CAD build for the part. Positions are in the model's coordinates, mm. Give positions to 0.01 mm unless a question says otherwise; leave off trailing zeros. Answer as a JSON object with one key per item and string values.
Autodesk Inventor part; units mm, degrees
ref_plane "C1_XY" through (0, 0, 0) normal (0, 0, 1) x (1, 0, 0)
ref_plane "C1_YZ" through (0, 0, 0) normal (1, 0, 0) x (0, 1, 0)
ref_plane "C1_ZX" through (0, 0, 0) normal (0, 1, 0) x (0, 0, 1)
sketch "Sketch_1" plane through (0, 0, 0) normal (0, 0, 1) x (1, 0, 0)
  line L0 (-10, -7) -> (-8, -7)
  line L1 (-8, -7) -> (-8, -4)
  line L2 (-8, -4) -> (-7.0607, -4)
  line L3 (-7.0607, -4) -> (-4, -7.0607)
  line L4 (-4, -7.0607) -> (-4, -9.4804)
  line L5 (-4, -9.4804) -> (-3.7, -10)
  line L6 (-3.7, -10) -> (-4, -10.5196)
  line L7 (-4, -10.5196) -> (-4, -12.9393)
  line L8 (-4, -12.9393) -> (-7.0607, -16)
  line L9 (-7.0607, -16) -> (-8, -16)
  line L10 (-8, -16) -> (-8, -13)
  line L11 (-8, -13) -> (-10, -13)
  line L12 (-10, -13) -> (-10, -19)
  arc A0 (-10, -19) -> (-9, -20) centre (-9, -19) ccw
  line L13 (-9, -20) -> (-3, -20)
  line L14 (-3, -20) -> (-3, -18)
  line L15 (-3, -18) -> (-6, -18)
  line L16 (-6, -18) -> (-6, -17.0607)
  line L17 (-6, -17.0607) -> (-2.9393, -14)
  line L18 (-2.9393, -14) -> (-0.5196, -14)
  line L19 (-0.5196, -14) -> (0, -13.7)
  line L20 (0, -13.7) -> (0.5196, -14)
  line L21 (0.5196, -14) -> (2.9393, -14)
  line L22 (2.9393, -14) -> (6, -17.0607)
  line L23 (6, -17.0607) -> (6, -18)
  line L24 (6, -18) -> (3, -18)
  line L25 (3, -18) -> (3, -20)
  line L26 (3, -20) -> (9, -20)
  arc A1 (9, -20) -> (10, -19) centre (9, -19) ccw
  line L27 (10, -19) -> (10, -13)
  line L28 (10, -13) -> (8, -13)
  line L29 (8, -13) -> (8, -16)
  line L30 (8, -16) -> (7.0607, -16)
  line L31 (7.0607, -16) -> (4, -12.9393)
  line L32 (4, -12.9393) -> (4, -10.5196)
  line L33 (4, -10.5196) -> (3.7, -10)
  line L34 (3.7, -10) -> (4, -9.4804)
  line L35 (4, -9.4804) -> (4, -7.0607)
  line L36 (4, -7.0607) -> (7.0607, -4)
  line L37 (7.0607, -4) -> (8, -4)
  line L38 (8, -4) -> (8, -7)
  line L39 (8, -7) -> (10, -7)
  line L40 (10, -7) -> (10, 7)
  line L41 (10, 7) -> (8, 7)
  line L42 (8, 7) -> (8, 4)
  line L43 (8, 4) -> (7.0607, 4)
  line L44 (7.0607, 4) -> (4, 7.0607)
  line L45 (4, 7.0607) -> (4, 9.4804)
  line L46 (4, 9.4804) -> (3.7, 10)
  line L47 (3.7, 10) -> (4, 10.5196)
  line L48 (4, 10.5196) -> (4, 12.9393)
  line L49 (4, 12.9393) -> (7.0607, 16)
  line L50 (7.0607, 16) -> (8, 16)
  line L51 (8, 16) -> (8, 13)
  line L52 (8, 13) -> (10, 13)
  line L53 (10, 13) -> (10, 19)
  arc A2 (10, 19) -> (9, 20) centre (9, 19) ccw
  line L54 (9, 20) -> (3, 20)
  line L55 (3, 20) -> (3, 18)
  line L56 (3, 18) -> (6, 18)
  line L57 (6, 18) -> (6, 17.0607)
  line L58 (6, 17.0607) -> (2.9393, 14)
  line L59 (2.9393, 14) -> (0.5196, 14)
  line L60 (0.5196, 14) -> (0, 13.7)
  line L61 (0, 13.7) -> (-0.5196, 14)
  line L62 (-0.5196, 14) -> (-2.9393, 14)
  line L63 (-2.9393, 14) -> (-6, 17.0607)
  line L64 (-6, 17.0607) -> (-6, 18)
  line L65 (-6, 18) -> (-3, 18)
  line L66 (-3, 18) -> (-3, 20)
  line L67 (-3, 20) -> (-9, 20)
  arc A3 (-9, 20) -> (-10, 19) centre (-9, 19) ccw
  line L68 (-10, 19) -> (-10, 13)
  line L69 (-10, 13) -> (-8, 13)
  line L70 (-8, 13) -> (-8, 16)
  line L71 (-8, 16) -> (-7.0607, 16)
  line L72 (-7.0607, 16) -> (-4, 12.9393)
  line L73 (-4, 12.9393) -> (-4, 10.5196)
  line L74 (-4, 10.5196) -> (-3.7, 10)
  line L75 (-3.7, 10) -> (-4, 9.4804)
  line L76 (-4, 9.4804) -> (-4, 7.0607)
  line L77 (-4, 7.0607) -> (-7.0607, 4)
  line L78 (-7.0607, 4) -> (-8, 4)
  line L79 (-8, 4) -> (-8, 7)
  line L80 (-8, 7) -> (-10, 7)
  line L81 (-10, 7) -> (-10, -7)
  line L82 (-8, 1.7) -> (-8, -1.7)
  arc A4 (-8, -1.7) -> (-7.7, -2) centre (-7.7, -1.7) ccw
  line L83 (-7.7, -2) -> (-7.0636, -2)
  arc A5 (-6.8515, -2.0879) -> (-7.0636, -2) centre (-7.0636, -2.3) ccw
  line L84 (-6.8515, -2.0879) -> (-2.9393, -6)
  line L85 (-2.9393, -6) -> (2.9393, -6)
  line L86 (2.9393, -6) -> (6.8515, -2.0879)
  arc A6 (7.0636, -2) -> (6.8515, -2.0879) centre (7.0636, -2.3) ccw
  line L87 (7.0636, -2) -> (7.7, -2)
  arc A7 (7.7, -2) -> (8, -1.7) centre (7.7, -1.7) ccw
  line L88 (8, -1.7) -> (8, 1.7)
  arc A8 (8, 1.7) -> (7.7, 2) centre (7.7, 1.7) ccw
  line L89 (7.7, 2) -> (7.0636, 2)
  arc A9 (6.8515, 2.0879) -> (7.0636, 2) centre (7.0636, 2.3) ccw
  line L90 (6.8515, 2.0879) -> (2.9393, 6)
  line L91 (2.9393, 6) -> (-2.9393, 6)
  line L92 (-2.9393, 6) -> (-6.8515, 2.0879)
  arc A10 (-7.0636, 2) -> (-6.8515, 2.0879) centre (-7.0636, 2.3) ccw
  line L93 (-7.0636, 2) -> (-7.7, 2)
  arc A11 (-7.7, 2) -> (-8, 1.7) centre (-7.7, 1.7) ccw
extrude "Extrusion1" add sketch "Sketch_1" against normal blind 485
sketch "Sketch2" plane through (0, 0, -485) normal (0, 0, -1) x (-1, 0, 0)
  point P0 (0, 10)
hole "Hole1" at (0, 10, -485) direction (0, 0, 1) diameter 4.2 depth 485
pattern_linear "Rectangular Pattern1" count 2 spacing 20 along (0, -1, 0) of "Hole1"
ref_plane "C1_XY" through (0, 0, 0) normal (0, 0, 1) x (1, 0, 0)
ref_plane "C1_YZ" through (0, 0, 0) normal (1, 0, 0) x (0, 1, 0)
ref_plane "C1_ZX" through (0, 0, 0) normal (0, 1, 0) x (0, 0, 1)
properties part number "HFS5-2040-485"
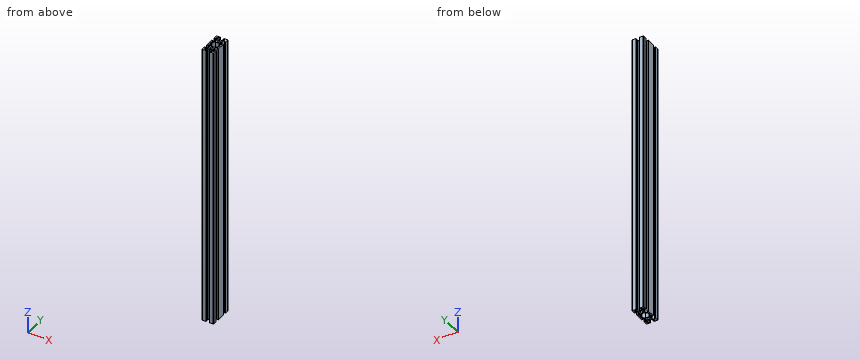
1) Slice it at A-A (z = -328). State how many separate pieces and enclosed holes the cut face has, then the cut area to 3 significant figures.
Model answer:
{"separate pieces": "1", "enclosed holes": "3", "area": "324 mm2"}
2) Wall check: probe 1 along Y at (x, z) = (0, -306.5); probe 2 along Y at (x, z) = (-5, -167); probe 3 along X at (y, z) = (10, -225). Give the ranges that are in metal, low to high.
Model answer:
{"probe 1": "y = -13.7 to -12.1, -7.9 to -6, 6 to 7.9, 12.1 to 13.7", "probe 2": "y = -20 to -18, -16.06 to -13.94, -6.06 to -3.94, 3.94 to 6.06, 13.94 to 16.06, 18 to 20", "probe 3": "x = -3.7 to -2.1, 2.1 to 3.7"}
3) Pin check, flat tips, straight feed: pin 1 (0.7 mm diameter, centred on x = -2, z = -252.5, fed in from +Y); pin 2 (4 mm diameter, centred on x = 0, z = -50, fed in from -Y); pin 3 (1.2 mm diameter, centred on y = -8.5, z = -179, fed in from -X). Stop position of each tip, or through.
Model answer:
{"pin 1": "stops at y = 14", "pin 2": "stops at y = -14", "pin 3": "stops at x = -4"}
